Build history of the part. All positions in model axes, mm. Round coordinates to 2 decimals unless told otherwise and drop trailing zeros. Loops run counter-clockwise (first coordinate to the right, second up) from the corner with the lowest first, then second, coordinate; pieces in that order, holes last. Notation, with made-up numbers: (34, 50.5) -> (66, 50.5) arc R17 cw to (66, 67.5) -> close; hole circle Ø8 at (-4, 88). An arc over 180 degrees is marked (long way). Put each result on its own line as item: value. Start each with the question number.
Item 1: Cut at A-A, the plane y = 4.5. List the corners of the cut face in (x, z).
Item 2: Flat gauge pins, fed straight in: pin 1 Ø2 at (y, z) = (-8.5, -72) entering from +X; pin 2 Ø4 at (y, z) = (-7, -15) entering from -X; pin 3 Ø3 at (x, y) = (149.5, 2.5) entering from +Z; pin 4 Ø10 at (x, z) = (139, -17.5) entering from +Y. Where does each tip first touch, or does it go through?
Item 3: Cut at C-C, the plane z = -17. Count the separate pieces of the cut face and the enclosed holes in it, plus the area to 3 significant figures.
Item 4: Cut at B-B, the plane x = 65. List the corners of the cut face in (y, z).
Item 5: Drill centre lines: probe 1 along Z at (x, y) = (2, 0); probe 2 along Z at (x, y) = (-70, 1); probe 3 along X at (y, z) = (6.75, -39.5). Where is each one in solid material? Low to high. Write a range as [from, to].
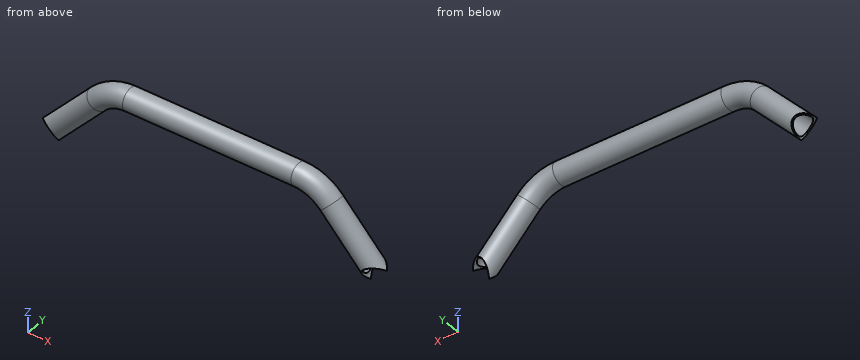
```python
from build123d import *
from build123d.topology import SkipClean

# Parameters (mm, degrees)
SKETCH_4_R          = 12.5
SKETCH_4_R_2        = 10.5
CUT_EXTRUDE_START   = -12.5000001
CUT_EXTRUDE_1_DEPTH = 25.0000001


# Read off the part's stored shape, not the designer's step: Вырез-Вытянуть1
with BuildPart() as part:
    # По траектории2: sweep along a path in Эскиз1
    with BuildLine(Plane(origin=(0, 0, 0), x_dir=(1, 0, 0), z_dir=(0, 1, 0))) as sweep_2_path:
        Line((-186.966101695, 73.672565631), (-132.818565926, 15.829831696))
        ThreePointArc((-132.818565926, 15.829831696), (-116.209877383, 4.127849745), (-96.316517235, 5.78e-07))
        Line((-96.316517235, 5.78e-07), (96.316517396, 5.78e-07))
        ThreePointArc((96.316517396, 5.78e-07), (116.209877578, 4.12784976), (132.818566138, 15.829831751))
        Line((132.818566138, 15.829831751), (186.966101695, 73.672565631))
    # Эскиз4 → По траектории2 (sweep)
    with BuildSketch(Plane(origin=(186.966101695, 0, -73.672565631), x_dir=(0.7300409748240902, 0, 0.6834033765485009), z_dir=(-0.6834033765485009, 0, 0.7300409748240902))):
        with Locations((0.952301131, 0)):
            Circle(SKETCH_4_R)
        with Locations((0.952301131, 0)):
            Circle(SKETCH_4_R_2, mode=Mode.SUBTRACT)
    sweep(path=sweep_2_path.line)

    # Вырез-Вытянуть1 outline → Вырез-Вытянуть1 (cut)
    with SkipClean():  # the faces are left unmerged after this step: merging them gives an invalid solid
        with BuildSketch(Plane(origin=(0, 0, 0), x_dir=(1, 0, 0), z_dir=(0, 1, 0)).offset(CUT_EXTRUDE_START)):
            with BuildLine():
                Line((196.786832727, 64.479217615), (178.535808357, 81.564302028))
                ThreePointArc((178.535808357, 81.564302028), (179.118778335, 63.896247636), (196.786832727, 64.479217615))
            make_face()
            with BuildLine():
                Line((-178.535808367, 81.564302042), (-196.786832713, 64.479217601))
                ThreePointArc((-196.786832713, 64.479217601), (-179.11877832, 63.896247649), (-178.535808367, 81.564302042))
            make_face()
        extrude(amount=CUT_EXTRUDE_1_DEPTH, mode=Mode.SUBTRACT)


solid = part.part
```
Reply:
1. outline: (-193.1, -61.77) arc R12.5 cw to (-189.02, -60.6) -> (-140.44, -8.7) arc R60.44 cw to (-96.32, 10.44) -> (96.32, 10.44) arc R60.44 cw to (140.44, -8.7) -> (189.02, -60.6) arc R12.5 cw to (193.1, -61.77) -> (142.03, -7.21) arc R62.61 ccw to (96.32, 12.61) -> (-96.32, 12.61) arc R62.61 ccw to (-142.03, -7.21) -> close; (-176.07, -77.71) -> (-125, -23.15) arc R39.29 cw to (-96.32, -10.71) -> (96.32, -10.71) arc R39.29 cw to (125, -23.15) -> (176.07, -77.71) arc R12.5 cw to (175.17, -73.56) -> (126.59, -21.66) arc R41.47 ccw to (96.32, -8.53) -> (-96.32, -8.53) arc R41.47 ccw to (-126.59, -21.66) -> (-175.17, -73.56) arc R12.5 cw to start
2. pin 1: stops at x = 175.33
2. pin 2: stops at x = -150.01
2. pin 3: stops at z = -12.68
2. pin 4: stops at y = 12.5
3. separate pieces: 2
3. enclosed holes: 2
3. area: 427 mm^2
4. outline: circle Ø25 at (0, 0.95); hole circle Ø21 at (0, 0.95)
5. probe 1: z = [-11.55, -9.55], [11.45, 13.45]
5. probe 2: z = [-11.51, -9.5], [11.4, 13.41]
5. probe 3: x = [-170.69, -167.3], [-145.26, -141.87], [141.87, 145.26], [167.3, 170.69]
